Can you work these out from the model? Positions are in its coordinate system, mm. A direction names the side the tool comes from. Round coordinates to 2 decimals unless told otherwise and drop trailing zeros. Loops run counter-clockwise (first coordinate to the right, second up) from the corner with the lowest first, then second, coordinate; pieces in that order, holes last. Notation, with made-up numbers: (-38, 2) -> (-17, 2) arc R34 cw to (-17, 36) -> close; hole circle Ø10 at (71.25, 81). An arc over 180 degrees is marked (long way). Use a Markdown table: item, result.
from build123d import *

# Parameters (mm, degrees)
SKETCH2_W           = 150
SKETCH2_H           = 150
BOSS_EXTRUDE1_DEPTH = 1300
SKETCH3_W           = 100
SKETCH3_H           = 50
CUT_EXTRUDE3_DEPTH  = 1150
SKETCH4_W           = 150
SKETCH4_H           = 30
CUT_EXTRUDE4_DEPTH  = 1150


with BuildPart() as part:
    # Sketch2 → Boss-Extrude1 (new body)
    with BuildSketch(Plane(origin=(0, 0, 0), x_dir=(1, 0, 0), z_dir=(0, 1, 0))):
        Rectangle(SKETCH2_W, SKETCH2_H)
    extrude(amount=BOSS_EXTRUDE1_DEPTH)

    # Sketch3 → Cut-Extrude3 (cut)
    with BuildSketch(Plane(origin=(0, 1300, 0), x_dir=(-1, 0, 0), z_dir=(0, 1, 0))):
        with Locations((0, -50)):
            Rectangle(SKETCH3_W, SKETCH3_H)
        with Locations((0, 50)):
            Rectangle(SKETCH3_W, SKETCH3_H)
    extrude(amount=-CUT_EXTRUDE3_DEPTH, mode=Mode.SUBTRACT)

    # Sketch4 → Cut-Extrude4 (cut)
    with BuildSketch(Plane(origin=(0, 1300, 0), x_dir=(-1, 0, 0), z_dir=(0, 1, 0))):
        with Locations((0, -60)):
            Rectangle(SKETCH4_W, SKETCH4_H)
        with Locations((0, 60)):
            Rectangle(SKETCH4_W, SKETCH4_H)
    extrude(amount=-CUT_EXTRUDE4_DEPTH, mode=Mode.SUBTRACT)


solid = part.part
1. Will these pins go through, and if not, where does the flat tip stop? pin 1 Ø12.5 at (x, y) = (-64, 705) entering from -Z; pin 2 Ø10 at (x, y) = (33.5, 944) entering from +Z; pin 3 Ø4 at (x, z) = (-24.5, 53) entering from +Y.
Answer sheet:
| item | result |
|---|---|
| pin 1 | stops at z = -45 |
| pin 2 | stops at z = 25 |
| pin 3 | stops at y = 150 |
2. Which directions (+Z, -Z, +X, -X, +Y, -Y) give clear straight access to the entire face, cutting with the end or side of a thin tool? Please do faces 4 (the flat face through (1, 733, 25)), 5 (the flat face through (63, 733, -45)), 6 (the flat face through (-50, 733, -35)).
Answer sheet:
| item | result |
|---|---|
| face 4 | +Z, +Y |
| face 5 | -Z, +X, -X, +Y |
| face 6 | -Z, +Y |
3. I need wall thicknesses on line 1 (X direction, y = 188.5, z = 42.5); line 2 (Y direction, x = -46.5, z = 53.5); line 3 (Z direction, x = 64.5, y = 765). Which ranges of each line are inside material? Lowest first, please.
Answer sheet:
| item | result |
|---|---|
| line 1 | x = -75 to -50, 50 to 75 |
| line 2 | y = 0 to 150 |
| line 3 | z = -45 to 45 |
4. If we mould it in two halves opening along X, with no side actions, what happens to faces 1 (the flat face through (-1, 1300, -1)), 2 (the flat face through (-50, 733, 35)), 3 (the flat face through (-75, 641, 1))? For each: +X half, -X half, draft (parallel to the pull), parting line (faces both ways), or undercut.
Answer sheet:
| item | result |
|---|---|
| face 1 | draft |
| face 2 | undercut |
| face 3 | -X half |
5. I want a section at C-C (z = 63). Please give me the cut outline in (x, y), plus the area to 3 significant figures.
Answer sheet:
| item | result |
|---|---|
| outline | (-75, 0) -> (75, 0) -> (75, 150) -> (-75, 150) -> close |
| area | 22,500 mm² |
6. I want a section at B-B (y = 180). Please give me the cut outline in (x, z), plus the area to 3 significant figures.
Answer sheet:
| item | result |
|---|---|
| outline | (-75, -45) -> (-50, -45) -> (-50, -25) -> (50, -25) -> (50, -45) -> (75, -45) -> (75, 45) -> (50, 45) -> (50, 25) -> (-50, 25) -> (-50, 45) -> (-75, 45) -> close |
| area | 9,500 mm² |
7. I want a section at A-A (x = -13). Please give me the cut outline in (y, z).
Answer sheet:
| item | result |
|---|---|
| outline | (0, -75) -> (150, -75) -> (150, -25) -> (1300, -25) -> (1300, 25) -> (150, 25) -> (150, 75) -> (0, 75) -> close |
